Check sheet for the modelled part. Datum: model origin and axes. Units: mm. Give positions to 0.01 mm unless a question says otherwise; leave off trailing zeros. Order: outer loops, then holes, each group sorted by start corner. A loop starts at its lowest first (then second) coordinate and runs counter-clockwise, first axis right, second up.
```python
from build123d import *

# Parameters (mm, degrees)
SKETCH1_W           = 877.8875
SKETCH1_H           = 877.8875
SKETCH1_W_2         = 203.2
SKETCH1_H_2         = 203.2
BOSS_EXTRUDE1_DEPTH = 18.25625
CUT_EXTRUDE1_DEPTH  = 9.525


with BuildPart() as part:
    # Sketch1 → Boss-Extrude1 (new body)
    with BuildSketch(Plane(origin=(0, 0, 0), x_dir=(1, 0, 0), z_dir=(0, 1, 0))):
        Rectangle(SKETCH1_W, SKETCH1_H)
        with Locations((-235.74375, -184.94375)):
            Rectangle(SKETCH1_W_2, SKETCH1_H_2, mode=Mode.SUBTRACT)
    extrude(amount=BOSS_EXTRUDE1_DEPTH)

    # Sketch3 → Cut-Extrude1 (cut)
    with BuildSketch(Plane(origin=(0, 18.25625, 0), x_dir=(1, 0, 0), z_dir=(0, 1, 0))):
        Polygon((429.41875, 438.94375), (438.94375, 438.94375), (438.94375, -438.94375), (-438.94375, -438.94375), (-438.94375, 438.94375), (-429.41875, 438.94375), (-429.41875, -429.41875), (429.41875, -429.41875), align=None)
    extrude(amount=-CUT_EXTRUDE1_DEPTH, mode=Mode.SUBTRACT)


solid = part.part
```
(1) Thickness scan on L1, parallel to X at y = 5.25, z = 142; L2, parallel to X at y = 12.25, z = 220.5; L3, parallel to Z at x = -149, y = 5. Record the ranges inside material, lowest first.
(2) Sectioned sample at B-B (z = 231.5). Enter the section's corners in (x, y), plus the area to 3 significant figures.
(3) Go/stop test with flat-tipped pins: P1, Ø1, axis at y = 13.5, z = -216.5, coming from the -X side; P2, Ø10.5, axis at y = 15.5, z = -12.5, coming from the +X side; P3, Ø7.5, axis at x = -175.5, y = 15, coming from the +Z side. Record where each tip stops, or that it passes through.
(4) Sectioned sample at A-A (x = -275). Enter the section's corners in (y, z), plus the area to 3 significant figures.
(5) Sectioned sample at C-C (y = 4.25). Enter the section's corners in (x, z), plus the area to 3 significant figures.
Values follow:
1. L1: x = -438.94 to -337.34, -134.14 to 438.94
1. L2: x = -429.42 to -337.34, -134.14 to 429.42
1. L3: z = -438.94 to 83.34, 286.54 to 438.94
2. outline: (-438.94, 0) - (-337.34, 0) - (-337.34, 18.26) - (-429.42, 18.26) - (-429.42, 8.73) - (-438.94, 8.73) - close; (-134.14, 0) - (438.94, 0) - (438.94, 8.73) - (429.42, 8.73) - (429.42, 18.26) - (-134.14, 18.26) - close
2. area: 12,100 mm2
3. P1: stops at x = -429.42
3. P2: stops at x = 429.42
3. P3: stops at z = 429.42
4. outline: (0, -438.94) - (18.26, -438.94) - (18.26, 83.34) - (0, 83.34) - close; (0, 286.54) - (18.26, 286.54) - (18.26, 429.42) - (8.73, 429.42) - (8.73, 438.94) - (0, 438.94) - close
4. area: 12,200 mm2
5. outline: (-438.94, -438.94) - (438.94, -438.94) - (438.94, 438.94) - (-438.94, 438.94) - close; hole (-337.34, 83.34) - (-134.14, 83.34) - (-134.14, 286.54) - (-337.34, 286.54) - close
5. area: 729,000 mm2
